Model file for the job. Use its own axes, mm. Round coordinates to 2 decimals unless told otherwise and drop trailing zeros. Order: outer loops, then holes, each group sorted by start corner. A loop starts at its lowest first (then second) coordinate and runs counter-clockwise, first axis right, second up. Notation, with made-up numbers: (69.5, 52) - (78.5, 52) arc R22 ccw to (78.5, 82) - close; hole circle Ø8 at (-20, 61). An arc over 180 degrees is marked (long way). Answer as CSV lines item,"result". Start each with the question number.
1. Wall check: line 1 along X through (y, z) = (-0.6, -63.5); line 2 along X through (y, z) = (-0.05, 58); line 3 along Z through (x, y) = (2.5, -0.25). Give the ranges that are in metal, low to high. Write a range as [from, to].
2. Pin check, flat tips, straight feed: pin 1 Ø0.7 at (y, z) = (0.5, 47.5) entering from +X; pin 2 Ø0.7 at (x, y) = (306.5, 0) entering from -Z; pin 3 Ø1.1 at (x, y) = (-315.5, 0.5) entering from +Z. Stop position of each tip, or through.
3. Band-saw the part on A-A on x = 19.5. List the corners of the cut face in (y, z).
```python
from build123d import *

# Parameters (mm, degrees)
SKETCH1_W           = 635.3556
SKETCH1_H           = 145.542
BOSS_EXTRUDE1_DEPTH = 1.143
BOSS_EXTRUDE2_DEPTH = 3.175
SKETCH3_W           = 3.175
SKETCH3_H           = 38.1
CUT_EXTRUDE1_DEPTH  = 327.637727957
SKETCH4_W           = 2.3368
SKETCH4_H           = 72.771
CUT_EXTRUDE2_DEPTH  = 327.637727957


with BuildPart() as part:
    # Sketch1 → Boss-Extrude1 (new, symmetric)
    with BuildSketch(Plane(origin=(0, 0, 0), x_dir=(1, 0, 0), z_dir=(0, 1, 0))):
        Rectangle(SKETCH1_W, SKETCH1_H)
    extrude(amount=BOSS_EXTRUDE1_DEPTH, both=True)

    # Sketch2 → Boss-Extrude2 (add)
    with BuildSketch(Plane(origin=(0, 0, -72.771), x_dir=(-1, 0, 0), z_dir=(0, 0, -1))):
        Polygon((-284.8269005, -1.143), (-30.826511563, -1.143), (-30.822511063, 1.143), (-284.8229, 1.143), align=None)
        Polygon((30.8188995, -1.143), (284.819288437, -1.143), (284.823288937, 1.143), (30.8229, 1.143), align=None)
    extrude(amount=BOSS_EXTRUDE2_DEPTH)

    # Sketch3 → Cut-Extrude1 (cut, through all)
    with BuildSketch(Plane.XZ.offset(1.143)):
        with Locations((-316.0903, 53.721)):
            Rectangle(SKETCH3_W, SKETCH3_H)
    cut_extrude1 = extrude(amount=-CUT_EXTRUDE1_DEPTH, mode=Mode.SUBTRACT)

    # Mirror1: Cut-Extrude1 across plane
    add(cut_extrude1.mirror(Plane(origin=(0, 0, 0), x_dir=(0, 0, 1), z_dir=(1, 0, 0))), mode=Mode.SUBTRACT)

    # Sketch4 → Cut-Extrude2 (cut, through all)
    with BuildSketch(Plane.XZ.offset(1.143)):
        with Locations((0.0254, -36.3855)):
            Rectangle(SKETCH4_W, SKETCH4_H)
    extrude(amount=-CUT_EXTRUDE2_DEPTH, mode=Mode.SUBTRACT)


solid = part.part
```
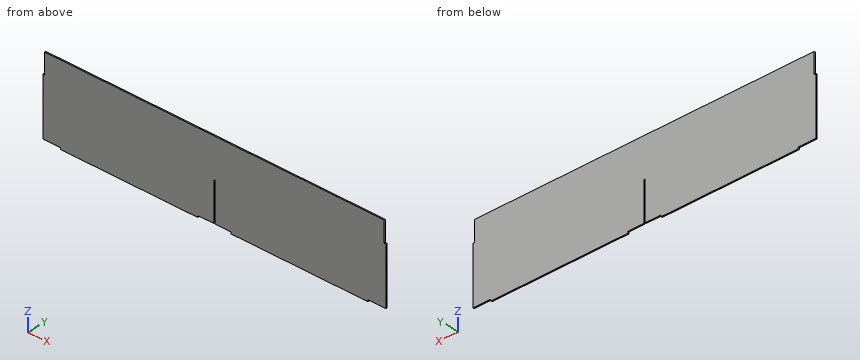
Reply:
1,line 1,"x = [-317.68, -1.14], [1.19, 317.68]"
1,line 2,"x = [-314.5, 314.5]"
1,line 3,"z = [-72.77, 72.77]"
2,pin 1,"stops at x = 314.5"
2,pin 2,"stops at z = -72.77"
2,pin 3,"stops at z = 34.67"
3,outline,"(-1.14, -72.77) - (1.14, -72.77) - (1.14, 72.77) - (-1.14, 72.77) - close"
